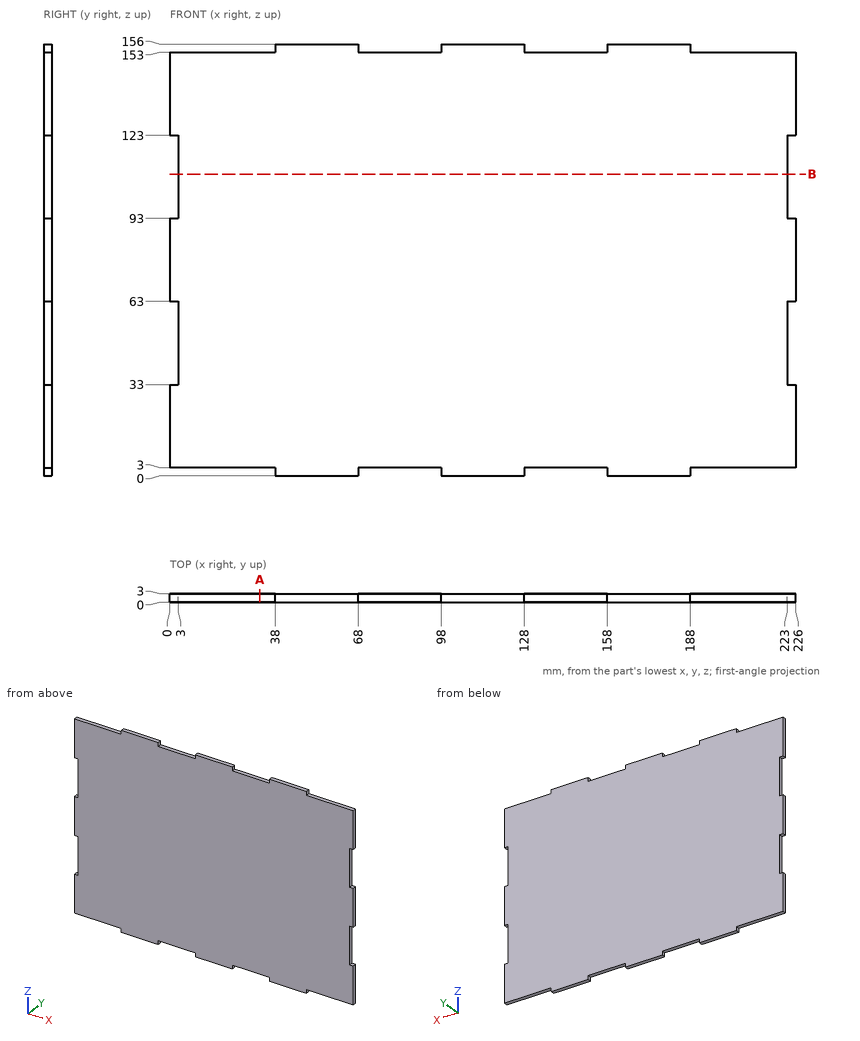
Study the drawing (mm; zero at the part's minimum x, y, z) and answer. Coordinates: 2 decimals unless noted, no trailing zeros. Loops run counter-clockwise (first coordinate to the right, second up) from the corner with the lowest first, then second, coordinate; pieces in that order, holes last. Notation, with made-up numbers: M 32,58 L 60,58 A7 ccw 60,64 Z; hole C 52,-30.75 d8. An arc over 180 degrees is marked long. Answer in a Markdown table with one row per item. Add a question column.
1. Consider L1, parallel to Z at x = 73, y = 1.15; L2, parallel to X at y = 1.05, z = 116. Determine where each line is inside the solid, lowest interval first.
2. Find section A-A, the plane x = 32.5. Write down the section's boundary in (y, z).
3. Flat-ended cylindrical pins translate along their axes: P1, Ø1.5, axis at y = 2, z = 154.5, coming from the -X side; P2, Ø1.5, axis at y = 1, z = 53.5, coming from the -X side; P3, Ø1, axis at x = 195.5, y = 1.5, coming from the +Z side. Find the tip coordinate at first contact, or state that the pin passes through.
4. Find section B-B, the plane z = 109. Write down the section's boundary in (x, y).
Reported:
| question | item | result |
|---|---|---|
| 1 | L1 | z = 3 to 153 |
| 1 | L2 | x = 3 to 223 |
| 2 | outline | M 0,3 L 3,3 L 3,153 L 0,153 Z |
| 3 | P1 | stops at x = 38 |
| 3 | P2 | stops at x = 3 |
| 3 | P3 | stops at z = 153 |
| 4 | outline | M 3,0 L 223,0 L 223,3 L 3,3 Z |
